```python
from build123d import *

# Parameters (mm, degrees)
SKETCH1_R           = 250
BOSS_EXTRUDE1_DEPTH = 900
CUT_EXTRUDE1_START  = -100
SKETCH5_R           = 200
CUT_EXTRUDE1_DEPTH  = 700
SKETCH6_R           = 65
CUT_EXTRUDE2_DEPTH  = 1356


with BuildPart() as part:
    # Sketch1 → Boss-Extrude1 (new body)
    with BuildSketch(Plane(origin=(0, 0, 0), x_dir=(1, 0, 0), z_dir=(0, 1, 0))):
        Circle(SKETCH1_R)
    extrude(amount=BOSS_EXTRUDE1_DEPTH)

    # Sketch5 → Cut-Extrude1 (cut)
    with BuildSketch(Plane(origin=(0, 0, 0), x_dir=(-1, 0, 0), z_dir=(0, -1, 0)).offset(CUT_EXTRUDE1_START)):
        Circle(SKETCH5_R)
    extrude(amount=-CUT_EXTRUDE1_DEPTH, mode=Mode.SUBTRACT)

    # Sketch6 → Cut-Extrude2 (cut)
    with BuildSketch(Plane(origin=(0, 900, 0), x_dir=(1, 0, 0), z_dir=(0, 1, 0))):
        Circle(SKETCH6_R)
    extrude(amount=-CUT_EXTRUDE2_DEPTH, mode=Mode.SUBTRACT)


solid = part.part
```
The model under review builds one solid part; all positions refer to its coordinate system, in mm. A direction names the side the tool comes from. Coordinates: 2 decimals unless noted, no trailing zeros. Write each loop counter-clockwise with the first axis right and the second up, starting at its lowest first coordinate (ties: lowest second). Pieces come first, ordered by that corner, then holes.
1) Clearance check with flat-ended pins moving along their axes: pin 1 Ø1 at (y, z) = (221, 138) entering from +X; pin 2 Ø6 at (x, y) = (148.5, 617.5) entering from +Z; pin 3 Ø2 at (y, z) = (124.5, 100.5) entering from -X. State where each tip first meets the part, or that it passes through.
2) To check wall thickness, follow probe 1 along Y at (x, z) = (-100.5, 134.5); probe 2 along X at (y, z) = (846, 0). State the ranges of each line that lie inside material, in increasing order.
3) The part is to be moulded in two halves that separate along X. For faces 1 (the face through (47, 100, -47)), 2 (the face through (-249.76, 443.7, -10.99)), 3 (the face through (52, 0, 52)), say which applies: pulls with the +X half, pulls with the -X half, needs draft (parallel to the pull), parting line crosses it, or undercut.
4) We need section A-A on x = 0. State the section outline as (y, z) points.
5) Machinability: for faces 4 (the face through (47, 800, -47)), 5 (the face through (62, 850.7, -19.52)), which of the approach directions +Z, -Z, +X, -X, +Y, -Y give a long, thin tool a straight path to every point of the face, cutting with its end or side? Answer none if there is none.
6) We need section C-C on z = 92. State the section outline as (x, y) points, then the cut area to 3 significant figures.
7) We need section B-B on z = 0. State the section outline as (x, y) points.
8) We need section D-D on x = 75. State the section outline as (y, z) points.
Answer list:
1. pin 1: stops at x = 208.79
1. pin 2: stops at z = 203.3
1. pin 3: stops at x = -229.35
2. probe 1: y = 0 to 100, 800 to 900
2. probe 2: x = -250 to -65, 65 to 250
3. face 1: undercut
3. face 2: parting line crosses it
3. face 3: needs draft
4. outline: (0, -250) - (900, -250) - (900, -65) - (800, -65) - (800, -200) - (100, -200) - (100, -65) - (0, -65) - close; (0, 65) - (100, 65) - (100, 200) - (800, 200) - (800, 65) - (900, 65) - (900, 250) - (0, 250) - close
5. face 4: none
5. face 5: +Y, -Y
6. outline: (-232.46, 0) - (232.46, 0) - (232.46, 900) - (-232.46, 900) - close; hole (-177.58, 100) - (177.58, 100) - (177.58, 800) - (-177.58, 800) - close
6. area: 170,000 mm2
7. outline: (-250, 0) - (-65, 0) - (-65, 100) - (-200, 100) - (-200, 800) - (-65, 800) - (-65, 900) - (-250, 900) - close; (65, 0) - (250, 0) - (250, 900) - (65, 900) - (65, 800) - (200, 800) - (200, 100) - (65, 100) - close
8. outline: (0, -238.48) - (900, -238.48) - (900, 238.48) - (0, 238.48) - close; hole (100, -185.4) - (800, -185.4) - (800, 185.4) - (100, 185.4) - close
